Here's the drawing with two shaded views (mm, measured from the low corner). I have some questions. A direction names the side the tool comes from. Give positions to 0.01 mm unless a question says otherwise; leave off trailing zeros. Loops run counter-clockwise (first coordinate to the right, second up) from the corner with the lowest first, then second, coordinate; pieces in that order, holes last. Notation, with made-up numbers: (-37, 25.25) -> (-11, 25.25) arc R18 ccw to (-11, 59.25) -> close; hole circle Ø2 at (-35.75, 43.25). An arc over 180 degrees is marked (long way). Answer in a Markdown table with one row per item. Add a question column.
Item 1: If we section it at A-A (z = 96): Write out the boundary of the cut face in (x, y), then the cut area to 3 significant figures.
Item 2: If I drill on line 1 (Z direction, x = 49, y = 75); line 2 (Y direction, x = 65, z = 78.5), over which ranges is the centre line in solid material (lowest first)?
Item 3: If we section it at C-C (y = 29): Write out the boundary of the cut face in (x, z).
Item 4: For P1, Ø23, axis at x = 85.5, z = 125, coming from the -Y side; P2, Ø23, axis at x = 69, z = 137, coming from the +Y side; P3, Ø1.5, axis at y = 16, z = 117.5, coming from the -X side; P4, Ø5, axis at x = 42.5, y = 13, coming from the +Z side, each with a flat end and sliding along its axis, tell me the tip position at first contact or that it passes through.
Item 5: Which directions (+Z, -Z, +X, -X, +Y, -Y) give clear straight access to the entire face, cutting with the end or side of a thin tool? Please do the marked faces 1, 2 and 3.
Item 6: If we section it at B-B (x = 49): Write out the boundary of the cut face in (y, z), then the cut area to 3 significant figures.
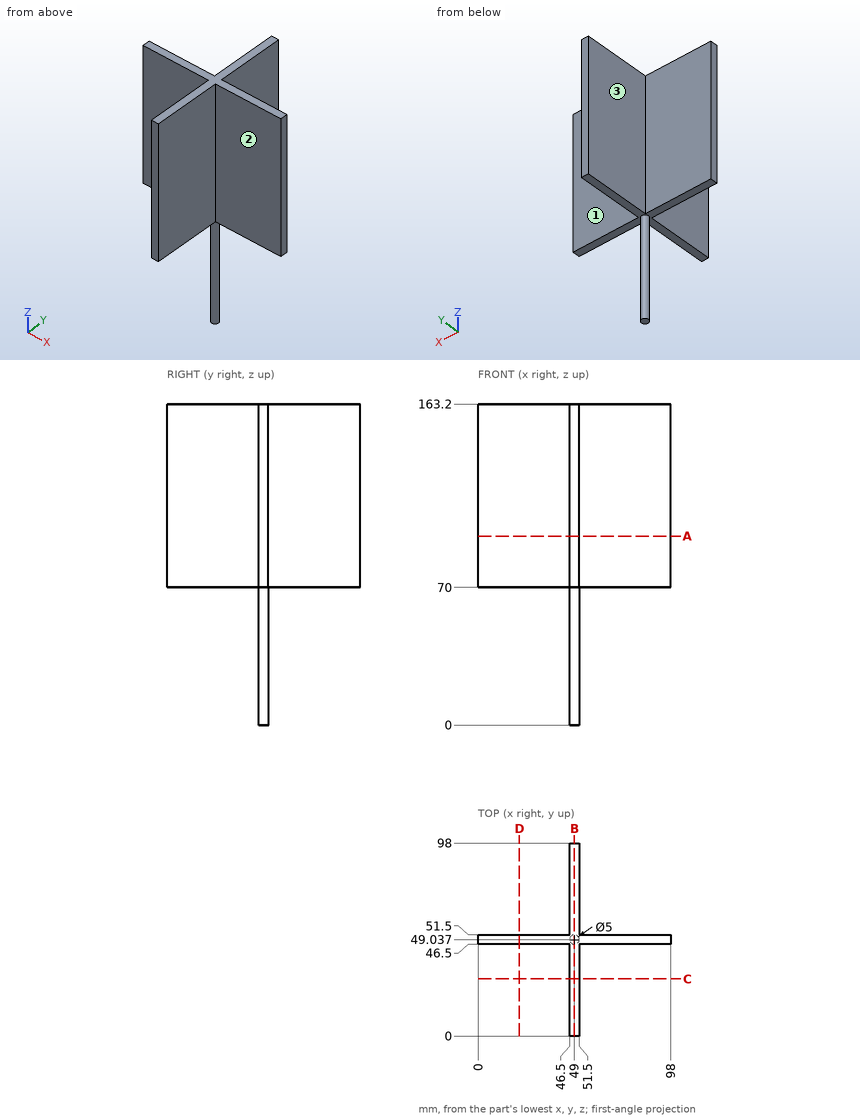
Recorded:
| question | item | result |
|---|---|---|
| 1 | outline | (0, 46.5) -> (46.5, 46.5) -> (46.5, 0) -> (51.5, 0) -> (51.5, 46.5) -> (98, 46.5) -> (98, 51.5) -> (51.5, 51.5) -> (51.5, 98) -> (46.5, 98) -> (46.5, 51.5) -> (0, 51.5) -> close |
| 1 | area | 955 mm^2 |
| 2 | line 1 | z = 70 to 163.2 |
| 2 | line 2 | y = 46.5 to 51.5 |
| 3 | outline | (46.5, 70) -> (51.5, 70) -> (51.5, 163.2) -> (46.5, 163.2) -> close |
| 4 | P1 | stops at y = 46.5 |
| 4 | P2 | stops at y = 51.5 |
| 4 | P3 | stops at x = 46.5 |
| 4 | P4 | passes through |
| 5 | face 1 | +Z, -Z, +X, +Y |
| 5 | face 2 | +Z, -Z, +X, -Y |
| 5 | face 3 | +Z, -Z, -X, +Y |
| 6 | outline | (0, 70) -> (46.54, 70) -> (46.54, 0) -> (51.54, 0) -> (51.54, 70) -> (98, 70) -> (98, 163.2) -> (0, 163.2) -> close |
| 6 | area | 9,480 mm^2 |
